```python
from build123d import *

# Parameters (mm, degrees)
F0_R      = 3.45
F1_DEPTH  = 17.5
F1_FACE_R = 3.45
F3_DEPTH  = 4.5
F2_R      = 4.7625
F2_R_2    = 3.45
F4_DEPTH  = 4.5
F5_R      = 10.65
F5_R_2    = 4.7625
F6_DEPTH  = 2
F7_R      = 2.95
F8_DEPTH  = 28


with BuildPart() as f1:
    # F0 (on Front) → F1 (new body)
    with BuildSketch(Plane.XZ):
        Circle(F0_R)
    extrude(amount=F1_DEPTH)

    # F1_face (on face) → F3 (join)
    with BuildSketch(Plane(origin=(0, 0, 0), x_dir=(1, 0, 0), z_dir=(0, 1, 0))):
        Circle(F1_FACE_R)
    extrude(amount=F3_DEPTH)

    # F2 (on face) → F4 (join)
    with BuildSketch(Plane(origin=(0, 0, 0), x_dir=(-1, 0, 0), z_dir=(0, 1, 0))):
        Circle(F2_R)
        Circle(F2_R_2, mode=Mode.SUBTRACT)
    extrude(amount=F4_DEPTH)

    # F5 (on face) → F6 (join)
    with BuildSketch(Plane(origin=(0, 4.5, 0), x_dir=(-1, 0, 0), z_dir=(0, 1, 0))):
        Circle(F5_R)
        Circle(F5_R_2, mode=Mode.SUBTRACT)
        Circle(F5_R_2)
    extrude(amount=F6_DEPTH)

    # F7 (on face) → F8 (cut)
    with BuildSketch(Plane.XZ.offset(17.5)):
        Circle(F7_R)
    extrude(amount=-F8_DEPTH, mode=Mode.SUBTRACT)


solid = f1.part
```
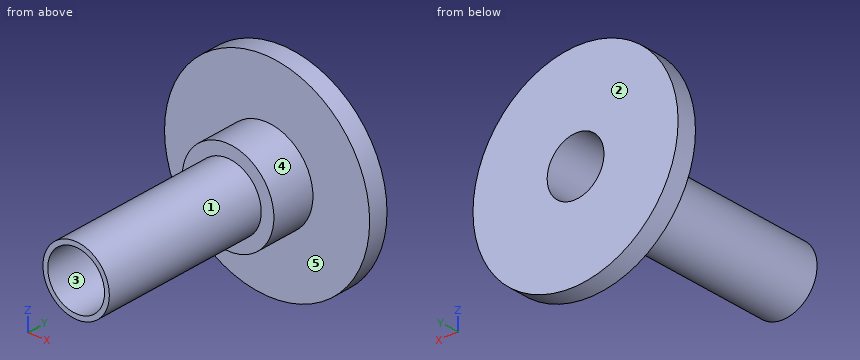
CAD build for the part. Positions are in the model's coordinates, mm. Face numbers are marked on the shaded views. A direction names the side the tool comes from. Round coordinates to 2 decimals unless told otherwise and drop trailing zeros. Loops run counter-clockwise (first coordinate to the right, second up) from the corner with the lowest first, then second, coordinate; pieces in that order, holes last. Notation, with made-up numbers: M 34,-19.75 L 82,-19.75 A16 ccw 82,5.25 Z; hole C 58.5,37.25 d10. An arc over 180 degrees is marked long. Use a Markdown table: item, result. Add a question column.
(1) Cut at D-D (z = -7.75). Give the cut face in (x, y), and give its area (3 significant figures).
(2) Cut at B-B (z = 1.5). Give the cut face in (x, y), and give its area (3 significant figures).
(3) Which spindle directions (+Z, -Z, +X, -X, +Y, -Y) get a long thin tool onto all of the face, cutting with end or side? Do the marked faces 1 and 2. Say none if no direction does.
(4) Cut at C-C (y = -10). Give the cut face in (x, z).
(5) Drill centre lines: line 1 (Z direction, x = 0, y = -7.5); line 2 (Y direction, x = 0.25, z = 4); line 3 (Y direction, x = 1.75, z = 4.5). Where is each one in solid material? Low to high.
(6) Cut at A-A (x = 0). Give the cut face in (y, z), and give its area (3 significant figures).
(7) Flat gauge pins, fed straight in: pin 1 (5 mm diameter, centred on y = -10, z = 4, fed in from +X); pin 2 (10 mm diameter, centred on x = 7.5, z = -7.5, fed in from -Y); pin 3 (6 mm diameter, centred on x = -7, y = -7, fed in from +Z); pin 4 (2 mm diameter, centred on x = -0.5, y = -13.5, fed in from -Z). Where does each tip first touch, or does it go through?
(8) Pull direction Z, two halves, no side cores. Call the marked faces 3, 4 and 5: +Z half, -Z half, draft (parallel to the pull), parting line (faces both ways), or undercut.
Geometry says:
| question | item | result |
|---|---|---|
| 1 | outline | M -7.3,4.5 L 7.3,4.5 L 7.3,6.5 L -7.3,6.5 Z |
| 1 | area | 29.2 mm² |
| 2 | outline | M -10.54,4.5 L -4.52,4.5 L -4.52,0 L -3.11,0 L -3.11,-17.5 L -2.54,-17.5 L -2.54,6.5 L -10.54,6.5 Z; M 2.54,-17.5 L 3.11,-17.5 L 3.11,0 L 4.52,0 L 4.52,4.5 L 10.54,4.5 L 10.54,6.5 L 2.54,6.5 Z |
| 2 | area | 69.7 mm² |
| 3 | face 1 | -Y |
| 3 | face 2 | +Z, -Z, +X, -X, +Y |
| 4 | outline | C 0,0 d6.9; hole C 0,0 d5.9 |
| 5 | line 1 | z = -3.45 to -2.95, 2.95 to 3.45 |
| 5 | line 2 | y = 0 to 6.5 |
| 5 | line 3 | y = 4.5 to 6.5 |
| 6 | outline | M -17.5,-3.45 L 0,-3.45 L 0,-4.76 L 4.5,-4.76 L 4.5,-10.65 L 6.5,-10.65 L 6.5,-2.95 L -17.5,-2.95 Z; M -17.5,2.95 L 6.5,2.95 L 6.5,10.65 L 4.5,10.65 L 4.5,4.76 L 0,4.76 L 0,3.45 L -17.5,3.45 Z |
| 6 | area | 64.6 mm² |
| 7 | pin 1 | stops at x = 3.11 |
| 7 | pin 2 | stops at y = 4.5 |
| 7 | pin 3 | passes through |
| 7 | pin 4 | stops at z = -3.45 |
| 8 | face 3 | undercut |
| 8 | face 4 | parting line |
| 8 | face 5 | draft |
